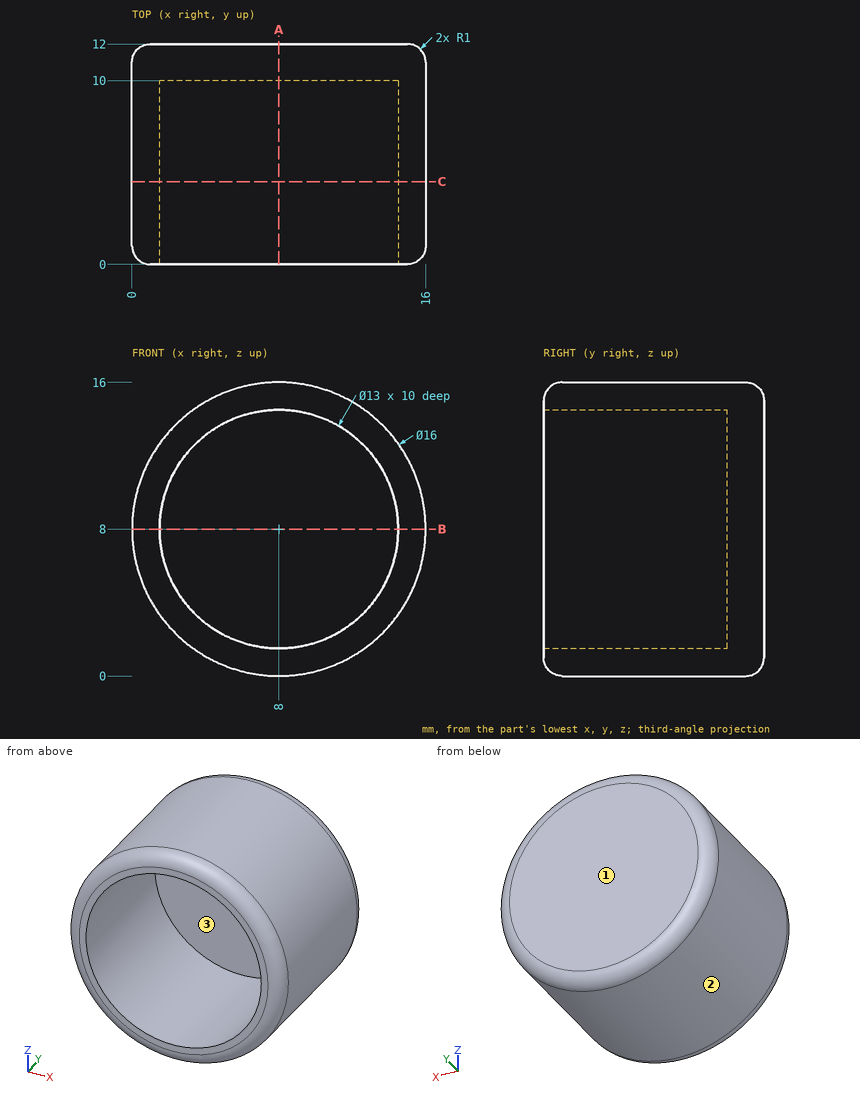
Verification items for this drawing (mm, ordinates from the low corner). Give positions to 0.01 mm unless a question says otherwise; leave off trailing zeros. Loops run counter-clockwise (first coordinate to the right, second up) from the corner with the lowest first, then second, coordinate; pieces in that order, holes last.
(1) Section check C-C on y = 4.5. Record the cut outline in (x, z).
From the geometry:
outline: circle Ø16 at (8, 8); hole circle Ø13 at (8, 8)
(2) Section check B-B on z = 8. Record the cut outline in (x, y).
From the geometry:
outline: (0, 1) arc R1 ccw to (1, 0) - (1.5, 0) - (1.5, 10) - (14.5, 10) - (14.5, 0) - (15, 0) arc R1 ccw to (16, 1) - (16, 11) arc R1 ccw to (15, 12) - (1, 12) arc R1 ccw to (0, 11) - close
(3) Section check A-A on x = 8. Record the cut outline in (y, z).
From the geometry:
outline: (0, 1) arc R1 ccw to (1, 0) - (11, 0) arc R1 ccw to (12, 1) - (12, 15) arc R1 ccw to (11, 16) - (1, 16) arc R1 ccw to (0, 15) - (0, 14.5) - (10, 14.5) - (10, 1.5) - (0, 1.5) - close
(4) Thickness scan on L1, parallel to Z at x = 8, y = 4; L2, parallel to Z at x = 5, y = 1.5; L3, parallel to Y at x = 10.75, z = 11.25. Record the ranges inside material, lowest first.
From the geometry:
L1: z = 0 to 1.5, 14.5 to 16
L2: z = 0.58 to 2.23, 13.77 to 15.42
L3: y = 10 to 12
(5) Release check for a two-part mould opening along X. For the marked faces 1, 2 and 3 record: released by +X, released by -X, zero draft, split by the parting line, or undercut.
From the geometry:
face 1: zero draft
face 2: split by the parting line
face 3: undercut
(6) Depth check by flat-ended pin: pin 1 Ø1 at (x, z) = (6.5, 2.5) entering from -Y; pin 2 Ø1.5 at (y, z) = (7.5, 13.5) entering from -X; pin 3 Ø4 at (x, y) = (7, 7.5) entering from -Z; pin 4 Ø1 at (x, y) = (4, 1.5) entering from +Z. Enter the tip coordinate at first touch or a pass-through.
From the geometry:
pin 1: stops at y = 10
pin 2: stops at x = 1.56
pin 3: stops at z = 0
pin 4: stops at z = 15.19
